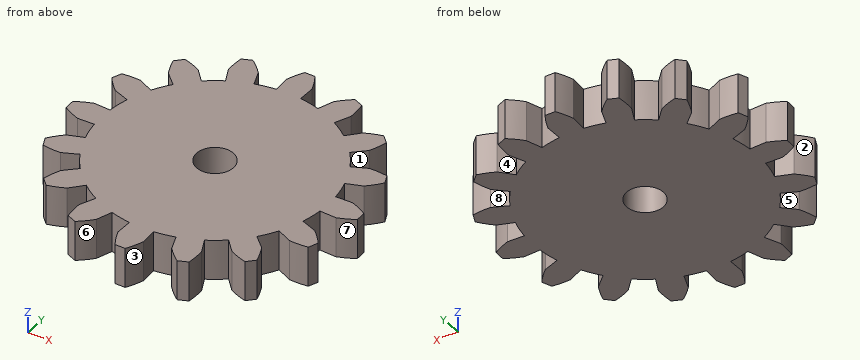
```python
from build123d import *

# Parameters (mm, degrees)
F0_R            = 17.78
F0_R_2          = 2.921
F1_DEPTH        = 6.35
F3_DEPTH        = 6.35
F3_COPIES_COUNT = 16


# Not quite as in the source:
# - a pattern or mirror of a feature is missing from the dataset's text; its kind, count and spacing are read off the source's solid


with BuildPart() as f1:
    # F0 (on Top) → F1 (new body)
    with BuildSketch(Plane.XY):
        Circle(F0_R)
        Circle(F0_R_2, mode=Mode.SUBTRACT)
    extrude(amount=F1_DEPTH)

    # F2 (on face) → F3 (join)
    with BuildSketch(Plane.XY.offset(6.35)):
        with BuildLine():
            Line((1.8639226102, 16.8154710155), (1.9928398674, 20.2606273541))
            ThreePointArc((1.9928398674, 20.2606273541), (1.461833226, 21.5784372569), (0.7936344478, 22.8322719293))
            Line((0.7936344478, 22.8322719293), (-0.0017393364, 22.8322719293))
            Line((-0.0017393364, 22.8322719293), (-0.7971131206, 22.8322719293))
            ThreePointArc((-0.7971131206, 22.8322719293), (-1.4653118988, 21.5784372569), (-1.9963185402, 20.2606273541))
            Line((-1.9963185402, 20.2606273541), (-1.8674012831, 16.8154710155))
            Line((-1.8674012831, 16.8154710155), (-0.0017393364, 16.8154710155))
            Line((-0.0017393364, 16.8154710155), (1.8639226102, 16.8154710155))
        make_face()
    f3 = extrude(amount=-F3_DEPTH)

    # F3_copies: F3 ×16 about axis
    f3_copies_axis = Axis((0, 0, 0), (0, 0, 1))
    for i in range(1, F3_COPIES_COUNT):
        add(f3.rotate(f3_copies_axis, i * 360 / F3_COPIES_COUNT))


solid = f1.part
```
For this review, take the finished solid that the model builds, in its own axes (mm). Face numbers are marked on the shaded views. A direction names the side the tool comes from. Round coordinates to 2 decimals unless told otherwise and drop trailing zeros. Write each loop counter-clockwise with the first axis right and the second up, starting at its lowest first coordinate (ties: lowest second). Pieces come first, ordered by that corner, then holes. Notation, with made-up numbers: (48, 44.5) -> (86, 44.5) arc R35 ccw to (86, 78.5) -> close; hole circle Ø3 at (45.5, 52). An arc over 180 degrees is marked (long way). One line per question, with ' | ' between items. Start each with the question number.
1) Add section A-A (y = 0). Write out the cut boundary in (x, z), and give its area (3 significant figures).
2) Wall thickness on line 1 along Y through (x, z) = (0, 2.75); line 2 along Y through (x, z) = (18, 4.25); line 3 along X through (y, z) = (-14, 2): over which ranges is each line inside the solid? List them lowest first.
3) Add section B-B (x = -14.5). Write out the cut boundary in (y, z).
4) Mouldability with a two-part tool opening along X and no side actions: class the marked faces 1, 2 and 3 as +X half, -X half, draft (parallel to the pull), parting line (faces both ways), or undercut.
5) Machinability: for the marked faces 4, 5, 6, 7 and 8, which of the approach directions +Z, -Z, +X, -X, +Y, -Y give a long, thin tool a straight path to every point of the face, cutting with its end or side? Answer none if there is none.
6) For pin 1 Ø1 at (x, z) = (-16, 4) entering from -Y; pin 2 Ø1.5 at (x, z) = (8, 3.5) entering from -Y, all flat-tipped, find the tip position at first contact; note any pin that passes through.
Reported:
1) outline: (-22.83, 0) -> (-2.92, 0) -> (-2.92, 6.35) -> (-22.83, 6.35) -> close; (2.92, 0) -> (22.83, 0) -> (22.83, 6.35) -> (2.92, 6.35) -> close | area: 253 mm²
2) line 1: y = -22.83 to -2.92, 2.92 to 22.83 | line 2: y = -9.6 to -5.36, -1.91 to 1.91, 5.36 to 9.6 | line 3: x = -16.21 to -11.3, -10.96 to 10.96, 11.31 to 16.21
3) outline: (-16.39, 0) -> (-11.77, 0) -> (-11.77, 6.35) -> (-16.39, 6.35) -> close; (-10.29, 0) -> (10.29, 0) -> (10.29, 6.35) -> (-10.29, 6.35) -> close; (11.77, 0) -> (16.39, 0) -> (16.39, 6.35) -> (11.77, 6.35) -> close
4) face 1: +X half | face 2: -X half | face 3: undercut
5) face 4: +Z, -Z, +Y | face 5: +Z, -Z, -X | face 6: +Z, -Z, -Y | face 7: +Z, -Z, +X | face 8: +Z, -Z
6) pin 1: stops at y = -16.71 | pin 2: stops at y = -21.4
